Part model, mm, in its own coordinate system. A direction names the side the tool comes from. Coordinates: 2 decimals unless noted, no trailing zeros. Loops run counter-clockwise (first coordinate to the right, second up) from the corner with the lowest first, then second, coordinate; pieces in that order, holes last. Notation, with made-up numbers: M 4,45.25 L 18,45.25 A28 cw 18,65.25 Z; hole C 79,23 d4. An arc over 180 degrees is marked long. Use a Markdown table: item, result. Add a question column.
1) Pull direction Z, two halves, no side cores. Call faces 4 (the flat face through (-2.948, 0.74, -1.305)), 5 (the flat face through (-2.948, 0.761, 1.293)), 6 (the cylindrical face through (9, 0, 2)), 7 (the flat face through (-4, -1.3, 1.3)): released by +Z, released by -Z, zero draft, split by the parting line, or undercut.
2) Pin check, flat tips, straight feed: pin 1 Ø1 at (x, z) = (3, -1) entering from +Y; pin 2 Ø1.5 at (x, z) = (11.5, 2.5) entering from +Y; pin 3 Ø1 at (x, z) = (-0.5, -2.5) entering from -Y. Stop position of each tip, or through.
3) Wall check: probe 1 along X at (y, z) = (3, -1); probe 2 along Y at (x, z) = (12.75, 1); probe 3 along Y at (x, z) = (-2, 1). Give the ranges that are in metal, low to high. Write a range as from..to.
4) Band-saw the part on A-A (x = -2.5). List the corners of the cut face in (y, z), plus the area to 3 significant figures.
5) Tool access for faces 1 (the flat face through (-2.948, -0.761, -1.293)), 2 (the flat face through (18, 0, 0)), 3 (the flat face through (0, 2, -2)): list every direction of +Z, -Z, +X, -X, +Y, -Y with a clear straight run to the whole face (end or side of a thin tool).
6) Band-saw the part on B-B (x = 6.5). List the corners of the cut face in (y, z).
Autodesk Inventor part; units mm, degrees
ref_plane "Work Plane1" through (29, 0, 0) normal (0, -1, 0) x (1, 0, 0)
ref_plane "YZ Plane" through (0, 0, 0) normal (1, 0, 0) x (0, 1, 0)
ref_plane "XZ Plane" through (0, 0, 0) normal (0, 1, 0) x (-1, 0, 0)
sketch "Rascunho1" plane through (0, 0, 0) normal (0, 0, 1) x (1, 0, 0)
  line L0 (-1, 0) -> (18, 0)
  line L1 (18, 0) -> (18, 2)
  line L2 (18, 2) -> (0.75, 2)
  line L3 (0.75, 2) -> (0.3205, 2)
  line L4 (0.3205, 2) -> (0, 2)
  line L5 (0, 2) -> (0, 3.5)
  line L6 (0, 3.5) -> (-4, 3.5)
  line L7 (-4, 3.5) -> (-4, 1.7321)
  line L8 (-4, 1.7321) -> (-2, 1.7321)
  line L9 (-2, 1.7321) -> (-1, 0)
  line L10 (-8.4, 0) -> (22.4, 0)
  line L11 (0, -0.7) -> (0, 4.2)
  line L12 (0.75, 2) -> (0, 2) construction
  dimension "d1" = 17.25
  dimension "d2" = 0.4295
  dimension "d3" = 4
  dimension "d4" = 2
  dimension "d5" = 60
  dimension "d6" = 4
  dimension "d7" = 4
  dimension "d8" = 3.4641
  dimension "d9" = 7
  dimension "d26" = 18
revolve "Corpo" add sketch "Rascunho1" angle 360 about axis through (-1, 0, 0) along (1, 0, 0)
sketch "Rascunho2" plane through (-4, 0, 0) normal (-1, 0, 0) x (0, 0, 1)
  circle A0 centre (0, 0) radius 1.7321
  line L0 (0, -4.9) -> (0, 4.9)
  line L1 (-4.9, 0) -> (4.9, 0)
  line L2 (1.7321, 0) -> (0.866, -1.5)
  line L3 (0.866, -1.5) -> (-0.866, -1.5)
  line L4 (-0.866, -1.5) -> (-1.7321, 0)
  line L5 (-1.7321, 0) -> (-0.866, 1.5)
  line L6 (-0.866, 1.5) -> (0.866, 1.5)
  line L7 (0.866, 1.5) -> (1.7321, 0)
extrude "Fenda" add sketch "Rascunho2" against normal up to next contours L7 A0 | A0 L2 | L6 L0 A0 | A0 L0 L3 | L0 L6 A0 | A0 L3 L0 | L4 A0 | A0 L5
fillet "Raio de arredondamento1" radius 0.4 1 edges at (-4, -3.5, 0)
thread "Rosca"
chamfer "Chanfrar1" distance 0.4294 distance2 0.4294 1 edges at (18, -2, 0) measured on face at (18, 0.527, -0.2661)
ref_plane "Work Plane1" through (29, 0, 0) normal (0, -1, 0) x (1, 0, 0)
fillet "Fillet2" radius 0.1 1 edges at (0, -2, 0)
equation "\"d1\" = GEL"
equation "\"d3\" = KOH"
equation "\"d4\" = INTI"
equation "\"d6\" = GD"
equation "\"d7\" = BDM"
equation "\"d8\" = 1.1547 * SW"
equation "\"d9\" = KOD"
equation "\"d26\" = NLG"
equation "\"d17\" = RR"
equation "\"d13\" = GEL"
equation "\"d15\" = -0.5 * SPD + 0.5 * GD"
equation "\"d16\" = GUL"
equation "\"d30\" = R"
equation "\"GD\" = NND"
equation "\"NLG\" = 18"
equation "\"GEL\" = 17.25"
equation "\"KOD\" = 7"
equation "\"KOH\" = 4"
equation "\"INTI\" = 2"
equation "\"GAL\" = 0.61345 * PTC"
equation "\"GUL\" = 0.61345 * PTC"
equation "\"BDM\" = NND"
equation "\"SW\" = 3"
equation "\"RR\" = 0.4"
equation "\"SPD\" = NND - 1.2269 * PTC"
equation "\"R\" = 0.1"
equation "\"TOA\" = 30deg"
equation "\"GD1\" = THREADDIA - 1.2269 * PTC"
equation "\"THREADDIA\" = 4"
equation "\"FAWI\" = 45deg"
equation "\"ANG\" = 120deg"
equation "\"PTC\" = 0.7"
equation "\"NND\" = 4"
equation "\"E0\" = 1.155 * SW"
properties part number "DIN 912 M4x18" material "Aço Inox AISI 304"
Entries:
| question | item | result |
|---|---|---|
| 1 | face 4 | undercut |
| 1 | face 5 | undercut |
| 1 | face 6 | split by the parting line |
| 1 | face 7 | zero draft |
| 2 | pin 1 | y = 1.94 |
| 2 | pin 2 | y = 0.97 |
| 2 | pin 3 | y = -2.87 |
| 3 | probe 1 | -4..0 |
| 3 | probe 2 | -1.73..1.73 |
| 3 | probe 3 | -3.35..-1.27, 1.27..3.35 |
| 4 | outline | C 0,0 d7; hole M -1.5,-0.87 L 0,-1.73 L 1.5,-0.87 L 1.5,0.87 L 0,1.73 L -1.5,0.87 Z |
| 4 | area | 30.7 mm2 |
| 5 | face 1 | -X |
| 5 | face 2 | +Z, -Z, +X, +Y, -Y |
| 5 | face 3 | +X |
| 6 | outline | C 0,0 d4 |
